Build history of the part. All positions in model axes, mm. Round coordinates to 2 decimals unless told otherwise and drop trailing zeros. Loops run counter-clockwise (first coordinate to the right, second up) from the corner with the lowest first, then second, coordinate; pieces in that order, holes last.
from build123d import *

# Parameters (mm, degrees)
BOSS_EXTRUDE1_DEPTH   = 5
CUT_EXTRUDE1_REACH    = 104.103
SKETCH2_R             = 1.5
BODY_MOVE_COPY1_ANGLE = 90
SKETCH19_R            = 2.25
SKETCH19_W            = 40.05
SKETCH19_H            = 21
CUT_EXTRUDE9_DEPTH    = 103.102889283


with BuildPart() as part:
    # Sketch1 → Boss-Extrude1 (new body)
    with BuildSketch(Plane(origin=(0, 0, 0), x_dir=(1, 0, 0), z_dir=(0, 1, 0))):
        with BuildLine():
            Line((80, -20), (0, -20))
            ThreePointArc((0, -20), (-20, 0), (0, 20))
            Line((0, 20), (80, 20))
            ThreePointArc((80, 20), (100, 0), (80, -20))
        make_face()
    extrude(amount=BOSS_EXTRUDE1_DEPTH)

    # Sketch2 → Cut-Extrude1 (cut, up to next)
    with BuildSketch(Plane(origin=(0, 5, 0), x_dir=(1, 0, 0), z_dir=(0, 1, 0)), mode=Mode.PRIVATE) as cut_extrude1_sk1:
        with Locations(Location((0.002, 7.999999875, 0), (0, 0, 270))):
            Circle(SKETCH2_R)
    cut_extrude1_tool1 = extrude(cut_extrude1_sk1.sketch, amount=-CUT_EXTRUDE1_REACH, mode=Mode.PRIVATE) & part.part
    # Sketch2 → Cut-Extrude1 (cut, up to next)
    with BuildSketch(Plane(origin=(0, 5, 0), x_dir=(1, 0, 0), z_dir=(0, 1, 0)), mode=Mode.PRIVATE) as cut_extrude1_sk2:
        with Locations(Location((0.002, -8.00000025, 0), (0, 0, 270))):
            Circle(SKETCH2_R)
    cut_extrude1_tool2 = extrude(cut_extrude1_sk2.sketch, amount=-CUT_EXTRUDE1_REACH, mode=Mode.PRIVATE) & part.part
    add(cut_extrude1_tool1.solids().sort_by_distance((0.002, 5, -8))[0], mode=Mode.SUBTRACT)
    add(cut_extrude1_tool2.solids().sort_by_distance((0.002, 5, 8))[0], mode=Mode.SUBTRACT)


with BuildPart() as part_1:
    # Body-Move/Copy1: moved
    add(part.part.rotate(Axis((0, 0, 0), (1, 0, 0)), BODY_MOVE_COPY1_ANGLE))

    # Sketch19 → Cut-Extrude9 (cut, through all)
    with BuildSketch(Plane.XY.offset(5)):
        with Locations((94.4, -5)):
            Circle(SKETCH19_R)
        with Locations(Location((94.4, 5, 0), (0, 0, 180))):
            Circle(SKETCH19_R)
        with Locations(Location((45.6, 5, 0), (0, 0, 180))):
            Circle(SKETCH19_R)
        with Locations((45.6, -5)):
            Circle(SKETCH19_R)
        with Locations((70, 0)):
            Rectangle(SKETCH19_W, SKETCH19_H)
    extrude(amount=-CUT_EXTRUDE9_DEPTH, mode=Mode.SUBTRACT)


with BuildPart() as part_2:
    # Body-Move/Copy5: moved
    add(part_1.part.moved(Location((-120, 0, 0))))


with BuildPart() as part_3:
    # Body-Move/Copy6: moved
    add(part_2.part.moved(Location((0, 0, -5))))


solid = part_3.part
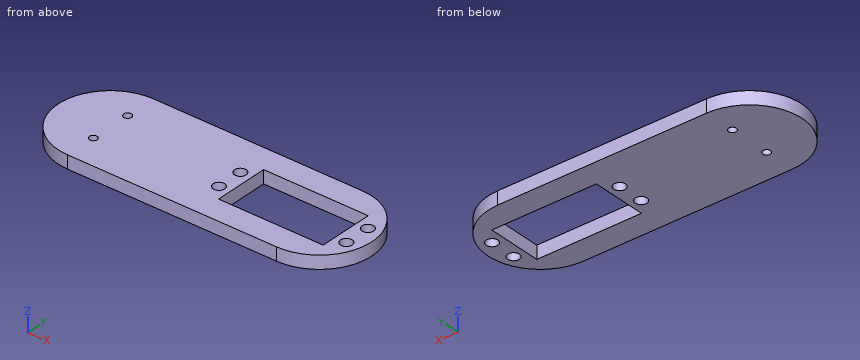
(1) Probe line 1 (Y direction, x = -74.4, z = -3.9); line 2 (X direction, y = 8, z = -1.9) (3 decimals); line 3 (X direction, y = 5.5, z = -1.4) (3 decimals). List the from-to ranges inside material, lowest first.
Responses:
line 1: y = -20 to -7.25, -2.75 to 2.75, 7.25 to 20
line 2: x = -138.33 to -121.498, -118.498 to -70.025, -29.975 to -21.67
line 3: x = -139.229 to -76.594, -72.206 to -70.025, -29.975 to -27.794, -23.406 to -20.771
(2) Slice it at C-C on x = -46.5. List the corners of the cut face in (y, z).
Responses:
outline: (-20, -5) - (-10.5, -5) - (-10.5, 0) - (-20, 0) - close; (10.5, -5) - (20, -5) - (20, 0) - (10.5, 0) - close
(3) Slice it at B-B on y = -5. List the corners of the cut face in (x, z) (3 decimals).
Responses:
outline: (-139.365, -5) - (-76.65, -5) - (-76.65, 0) - (-139.365, 0) - close; (-72.15, -5) - (-70.025, -5) - (-70.025, 0) - (-72.15, 0) - close; (-29.975, -5) - (-27.85, -5) - (-27.85, 0) - (-29.975, 0) - close; (-23.35, -5) - (-20.635, -5) - (-20.635, 0) - (-23.35, 0) - close
(4) Slice it at A-A on x = -74.4. List the corners of the cut face in (y, z).
Responses:
outline: (-20, -5) - (-7.25, -5) - (-7.25, 0) - (-20, 0) - close; (-2.75, -5) - (2.75, -5) - (2.75, 0) - (-2.75, 0) - close; (7.25, -5) - (20, -5) - (20, 0) - (7.25, 0) - close
(5) Slice it at D-D on z = -3.6. List the corners of the cut face in (x, y) (3 decimals).
Responses:
outline: (-120, -20) - (-40, -20) arc R20 ccw to (-40, 20) - (-120, 20) arc R20 ccw to start; hole circle Ø3 at (-119.998, -8); hole circle Ø3 at (-119.998, 8); hole circle Ø4.5 at (-74.4, -5); hole circle Ø4.5 at (-74.4, 5); hole (-70.025, -10.5) - (-29.975, -10.5) - (-29.975, 10.5) - (-70.025, 10.5) - close; hole circle Ø4.5 at (-25.6, -5); hole circle Ø4.5 at (-25.6, 5)
(6) Pin check, flat tip, straight feed: P1, Ø2.5, axis at y = 2.5, z = -2, coming from the -X side. Stop position of the tip, or through.
Responses:
P1: stops at x = -139.96
